The listing builds one solid part. Answer for the finished solid, in the listing's coordinates (mm). A direction names the side the tool comes from. Give positions to 0.01 mm unless a question says otherwise; leave off trailing zeros. Order: outer loops, then holes, each group sorted by start corner. A loop starts at its lowest first (then second) coordinate and runs counter-clockwise, first axis right, second up. Notation, with made-up numbers: (52, -17) - (75, -17) arc R21 ccw to (75, 12) - close; hole circle Ø8 at (87, 9.25). An arc over 180 degrees is marked (long way). Use CSV: the item, a comma, the result in double quotes.
```python
from build123d import *

# Parameters (mm, degrees)
PAD_DEPTH = 17


with BuildPart() as part:
    # Sketch → Pad (new body)
    with BuildSketch(Plane.XY):
        with BuildLine():
            Line((0, 17.5), (0, -15.248976))
            Line((-9.983073, -26.419536), (0, -15.248976))
            ThreePointArc((-9.983073, -26.419536), (-9.923619, -27.478522), (-8.864632, -27.41908))
            Line((0, -17.5), (-8.864632, -27.41908))
            Line((1, -17.5), (0, -17.5))
            Line((1, -15.25), (1, -17.5))
            Line((6, -18.136751), (1, -15.25))
            Line((6, -18.136751), (6, -23.5))
            Line((6, -23.5), (4.5, -23.5))
            Line((4.5, -23.5), (4.5, -29.5))
            Line((4.5, -29.5), (7.5, -29.5))
            Line((7.5, -29.5), (7.5, -31))
            Line((3, -31), (7.5, -31))
            Line((3, -20.5), (3, -31))
            Line((-0.669356, -20.5), (3, -20.5))
            Line((-10.5, -31.5), (-0.669356, -20.5))
            Line((-12.25, -31.5), (-10.5, -31.5))
            Line((-12.25, -29.75), (-12.25, -31.5))
            Line((-14, -29.75), (-12.25, -29.75))
            Line((-14, -31.5), (-14, -29.75))
            Line((-23.4282, -31.5), (-14, -31.5))
            ThreePointArc((-24.178201, -28.700962), (-24.877089, -30.388229), (-23.4282, -31.5))
            Line((-18.375, -25.350481), (-24.178201, -28.700962))
            ThreePointArc((-17.25, -26), (-17.625, -25.350481), (-18.375, -25.350481))
            Line((-17.25, -26), (-17.25, -26.75))
            Line((-15.5, -26.75), (-17.25, -26.75))
            Line((-15.5, -25.25), (-15.5, -26.75))
            Line((-12.961323, -25.25), (-15.5, -25.25))
            Line((-3, -14.103777), (-12.961323, -25.25))
            Line((-3, 21.500001), (-3, -14.103777))
            Line((-6.749997, 25.25), (-3, 21.500001))
            Line((-15.5, 25.25), (-6.749997, 25.25))
            Line((-15.5, 26.75), (-15.5, 25.25))
            Line((-17.25, 26.75), (-15.5, 26.75))
            Line((-17.25, 25.25), (-17.25, 26.75))
            Line((-21.5, 25.25), (-17.25, 25.25))
            Line((-21.5, 25.25), (-21.5, 28.25))
            Line((-21.5, 28.25), (-14, 28.25))
            Line((-14, 26.75), (-14, 28.25))
            Line((-12.25, 26.75), (-14, 26.75))
            Line((-12.25, 28.25), (-12.25, 26.75))
            Line((-12.25, 28.25), (-5.507356, 28.25))
            Line((-5.507356, 28.25), (6, 16.74264))
            Line((6, 16.74264), (6, 14.621319))
            Line((6, 14.621319), (3.87868, 14.621319))
            Line((3.87868, 14.621319), (1, 17.5))
            Line((1, 17.5), (0, 17.5))
        make_face()
    extrude(amount=PAD_DEPTH)


solid = part.part
```
Item 1: The part is cut by section A-A (x = -4). Give the vertices of the cut face in (y, z), and give its area (3 significant figures).
Taken from the geometry:
outline,"(-24.23, 0) - (-21.98, 0) - (-21.98, 17) - (-24.23, 17) - close; (-19.72, 0) - (-15.22, 0) - (-15.22, 17) - (-19.72, 17) - close; (22.5, 0) - (26.74, 0) - (26.74, 17) - (22.5, 17) - close"
area,"187 mm^2"
Item 2: Which of the six approach directions +Z, -Z, +X, -X, +Y, -Y give full straight-line access (tool end or side, diameter ignored) to faces 4 (the face through (6, -29.5, 8)), 5 (the face through (-11, 25.25, 8)), 6 (the face through (1, -16, 8)), 7 (the face through (-21.5, 27, 8)), 8 (the face through (-13, -29.75, 8))?
Taken from the geometry:
face 4,"+Z, -Z, +X"
face 5,"+Z, -Z, -X"
face 6,"+Z, -Z"
face 7,"+Z, -Z, -X, +Y"
face 8,"+Z, -Z, -Y"
Item 3: The part is cut by section D-D (y = 24.5). Give the vertices of the cut face in (x, z).
Taken from the geometry:
outline,"(-6, 0) - (-1.76, 0) - (-1.76, 17) - (-6, 17) - close"
Item 4: The part is cut by section C-C (y = -5). Give the vertices of the cut face in (x, z), and give its area (3 significant figures).
Taken from the geometry:
outline,"(-3, 0) - (0, 0) - (0, 17) - (-3, 17) - close"
area,"51.0 mm^2"
Item 5: The mould has two halves that part along Y. Classify faces 1 (the face through (-21.236, -27.002, 8.381)), 2 (the face through (3, -26, 8)), 3 (the face through (0.166, 22.577, 8.381)): +Y half, -Y half, draft (parallel to the pull), parting line (faces both ways), or undercut.
Taken from the geometry:
face 1,"undercut"
face 2,"draft"
face 3,"+Y half"
Item 6: Find the intervals of material crossed by line 1 along Y through (x, z) = (-6, 14.25); line 2 along Y through (x, z) = (-19.5, 13.75); line 3 along Y through (x, z) = (-13, 13.75), in increasing order.
Taken from the geometry:
line 1,"-26.46 to -24.21, -21.96 to -17.46, 24.5 to 28.25"
line 2,"-31.5 to -26, 25.25 to 28.25"
line 3,"-29.75 to -25.25, 25.25 to 26.75"
Item 7: The part is cut by section B-B (x = -19). Give the vertices of the cut face in (y, z).
Taken from the geometry:
outline,"(-31.5, 0) - (-25.71, 0) - (-25.71, 17) - (-31.5, 17) - close; (25.25, 0) - (28.25, 0) - (28.25, 17) - (25.25, 17) - close"
Item 8: Each of these flat-tipped pins is pushed along its axis until it touches: pin 1 (1.5 mm diameter, centred on y = 26, z = 5, fed in from -X); pin 2 (1.6 mm diameter, centred on y = -21, z = 4.5, fed in from +X); pin 3 (0.9 mm diameter, centred on x = -13.5, z = 10, fed in from +Y). Where does it stop, or does it pass through?
Taken from the geometry:
pin 1,"x = -21.5"
pin 2,"x = 6"
pin 3,"y = 26.75"
